Design review of the part built by this model. Coordinates are the model's own, in mm. A direction names the side the tool comes from. Give positions to 0.01 mm unless a question says otherwise; leave off trailing zeros. Write each loop counter-clockwise with the first axis right and the second up, starting at its lowest first coordinate (ties: lowest second). Pieces come first, ordered by that corner, then holes. Notation, with made-up numbers: M 77.25,39.25 L 98.25,39.25 A18 cw 98.25,43.25 Z; hole C -4.75,-20 d10. An arc over 180 degrees is marked long. Use a Markdown table: item, result. Add a question column.
```python
from build123d import *

# Parameters (mm, degrees)
EXTRUDE_1_DEPTH          = 46
EXTRUDE_1_DEPTH_BACK     = 46
EXTRUDE_2_DEPTH          = 41.75
EXTRUDE_2_DEPTH_BACK     = 41.75
CUT_EXTRUDE_1_DEPTH      = 40.75
CUT_EXTRUDE_1_DEPTH_BACK = 40.75
EXTRUDE_3_DEPTH          = 1
EXTRUDE_3_DEPTH_BACK     = 1
EXTRUDE_4_DEPTH          = 1
EXTRUDE_4_DEPTH_BACK     = 1
EXTRUDE_5_DEPTH          = 1
EXTRUDE_5_DEPTH_BACK     = 1
EXTRUDE_6_DEPTH          = 2
EXTRUDE_6_DEPTH_BACK     = 2
EXTRUDE_7_DEPTH          = 2
EXTRUDE_7_DEPTH_BACK     = 2


with BuildPart() as part:
    # 草图1 → 凸台-拉伸1 (new, two sides: drawn at the far end of the back side and taken through both)
    with BuildSketch(Plane.XY.offset(-EXTRUDE_1_DEPTH_BACK)):
        Polygon((-2, 41), (-2, 0), (0, 0), (0, 39.267949192), (-1, 41), align=None)
    extrude(amount=EXTRUDE_1_DEPTH + EXTRUDE_1_DEPTH_BACK)

    # 草图2 → 凸台-拉伸2 (add, two sides: drawn at the far end of the back side and taken through both)
    with BuildSketch(Plane.XY.offset(-EXTRUDE_2_DEPTH_BACK)):
        with BuildLine():
            Line((-23.15444772, 45.322915161), (-23, 23.723915946))
            Line((-23, 23.723915946), (-2, 6.102823691))
            Line((-2, 6.102823691), (-2, 37.107539179))
            Line((-2, 37.107539179), (-18.24692063, 47.968020382))
            ThreePointArc((-18.24692063, 47.968020382), (-21.496697605, 48.122330559), (-23.15444772, 45.322915161))
        make_face()
    extrude(amount=EXTRUDE_2_DEPTH + EXTRUDE_2_DEPTH_BACK)

    # 草图3 → 切除-拉伸1 (cut, two sides: drawn at the far end of the back side and taken through both)
    with BuildSketch(Plane.XY.offset(-CUT_EXTRUDE_1_DEPTH_BACK)):
        with BuildLine():
            Line((-22, 24.190223604), (0, 5.730031718))
            Line((0, 5.730031718), (0, 35.071545943))
            Line((0, 35.071545943), (-18.919301008, 47.184362345))
            ThreePointArc((-18.919301008, 47.184362345), (-20.957600798, 47.254585951), (-21.9976903, 45.500216772))
            Line((-21.9976903, 45.500216772), (-22, 24.190223604))
        make_face()
    extrude(amount=CUT_EXTRUDE_1_DEPTH + CUT_EXTRUDE_1_DEPTH_BACK, mode=Mode.SUBTRACT)

    # 草图4 → 凸台-拉伸3 (add, two sides: drawn at the far end of the back side and taken through both)
    with BuildSketch(Plane.XY.offset(-EXTRUDE_3_DEPTH_BACK)):
        Polygon((-8.210146219, 39.5), (-3.5, 37.303622747), (-3.5, 39.5), align=None)
    extrude(amount=EXTRUDE_3_DEPTH + EXTRUDE_3_DEPTH_BACK)

    # 草图6 → 凸台-拉伸4 (add, two sides: drawn at the far end of the back side and taken through both)
    with BuildSketch(Plane.XY.offset(-36.75).offset(-EXTRUDE_4_DEPTH_BACK)):
        Polygon((-8.210146219, 39.5), (-3.5, 37.303622747), (-3.5, 39.5), align=None)
    extrude(amount=EXTRUDE_4_DEPTH + EXTRUDE_4_DEPTH_BACK)

    # 草图5 → 凸台-拉伸5 (add, two sides: drawn at the far end of the back side and taken through both)
    with BuildSketch(Plane.XY.offset(36.75).offset(-EXTRUDE_5_DEPTH_BACK)):
        Polygon((-8.210146219, 39.5), (-3.5, 37.303622747), (-3.5, 39.5), align=None)
    extrude(amount=EXTRUDE_5_DEPTH + EXTRUDE_5_DEPTH_BACK)

    # 草图7 → 凸台-拉伸6 (add, two sides: drawn at the far end of the back side and taken through both)
    with BuildSketch(Plane.XY.offset(-36.75).offset(-EXTRUDE_6_DEPTH_BACK)):
        Polygon((-13.201666314, 16.207545053), (-3.5, 4.645549369), (-3.5, 8.066880427), align=None)
    extrude(amount=EXTRUDE_6_DEPTH + EXTRUDE_6_DEPTH_BACK)

    # 草图8 → 凸台-拉伸7 (add, two sides: drawn at the far end of the back side and taken through both)
    with BuildSketch(Plane.XY.offset(36.75).offset(-EXTRUDE_7_DEPTH_BACK)):
        Polygon((-13.201666314, 16.207545053), (-3.5, 4.645549369), (-3.5, 8.066880427), align=None)
    extrude(amount=EXTRUDE_7_DEPTH + EXTRUDE_7_DEPTH_BACK)


solid = part.part
```
(1) Wall thickness on L1, parallel to Z at x = -9.25, y = 27.5; L2, parallel to Z at x = -1.25, y = 31.5; L3, parallel to Y at x = -6.75, z = -28: over which ranges is each line inside the solid? List them lowest first.
(2) Add section C-C on y = 36. Give the boundary of the cut face in (x, z).
(3) The part is to be moulded in two halves that separate along Z. For faces 1 (the flat face through (-13, 28, 41.75)), 2 (the flat face through (-7.405, 9.299, 36.722)), 3 (the cylindrical face through (-20.93, 47.27, -0.57)), 4 (the flat face through (-11, 27, 40.75)), say which applies: released by +Z, released by -Z, zero draft, split by the parting line, or undercut.
(4) Add section D-D on y = 9.5. Give the boundary of the cut face in (x, z), then the cut area to 3 significant figures.
(5) Add section A-A on x = -14.25. Give the boundary of the cut face in (y, z).
(6) For pin 1 (12 mm diameter, centred on y = 26, z = 23, fed in from +X); pin 2 (12 mm diameter, centred on y = 12, z = -16.5, fed in from -X); pin 3 (10 mm diameter, centred on x = -7.5, y = 11, fed in from +Z), all flat-tipped, find the tip position at first contact; note any pin that passes through.
(7) Machinability: for faces 5 (the flat face through (-6, 9, 34.75)), 6 (the flat face through (-6, 9, 38.75)), 7 (the flat face through (-11.154, 15.089, -0.571)), which of the approach directions +Z, -Z, +X, -X, +Y, -Y give a long, thin tool a straight path to every point of the face, cutting with its end or side? Answer none if there is none.
(8) Add section B-B on z = -14.5. Give the boundary of the cut face in (x, y), then the cut area to 3 significant figures.
From the geometry:
| question | item | result |
|---|---|---|
| 1 | L1 | z = -41.75 to -40.75, 40.75 to 41.75 |
| 1 | L2 | z = -46 to -40.75, 40.75 to 46 |
| 1 | L3 | y = 10.09 to 11.39, 39.39 to 40.28 |
| 2 | outline | M -23.09,-41.75 L -2,-41.75 L -2,-46 L 0,-46 L 0,46 L -2,46 L -2,41.75 L -23.09,41.75 Z; hole M -22,-40.75 L -1.45,-40.75 L -1.45,40.75 L -22,40.75 Z |
| 3 | face 1 | released by +Z |
| 3 | face 2 | zero draft |
| 3 | face 3 | undercut |
| 3 | face 4 | undercut |
| 4 | outline | M -7.57,-38.75 L -6.05,-38.75 L -6.05,-41.75 L -2,-41.75 L -2,-46 L 0,-46 L 0,-40.75 L -4.49,-40.75 L -4.49,40.75 L 0,40.75 L 0,46 L -2,46 L -2,41.75 L -6.05,41.75 L -6.05,38.75 L -7.57,38.75 L -7.57,34.75 L -6.05,34.75 L -6.05,-34.75 L -7.57,-34.75 Z |
| 4 | area | 168 mm^2 |
| 5 | outline | M 16.38,-41.75 L 45.3,-41.75 L 45.3,41.75 L 16.38,41.75 Z; hole M 17.69,-40.75 L 44.19,-40.75 L 44.19,40.75 L 17.69,40.75 Z |
| 6 | pin 1 | stops at x = -17.01 |
| 6 | pin 2 | stops at x = -16.18 |
| 6 | pin 3 | stops at z = 41.75 |
| 7 | face 5 | -X, -Y |
| 7 | face 6 | +Z, -X, -Y |
| 7 | face 7 | +X |
| 8 | outline | M -23.15,45.32 L -23,23.72 L -2,6.1 L -2,0 L 0,0 L 0,5.73 L -22,24.19 L -22,45.5 A2 cw -18.92,47.18 L 0,35.07 L 0,39.27 L -1,41 L -2,41 L -2,37.11 L -18.25,47.97 A3.15 ccw Z |
| 8 | area | 95.0 mm^2 |
